Autodesk Inventor part; units mm, degrees
ref_plane "XZ Plane" through (0, 0, 0) normal (0, 1, 0) x (-1, 0, 0)
ref_plane "XY Plane" through (0, 0, 0) normal (0, 0, 1) x (1, 0, 0)
sketch "Sketch1" plane through (0, 0, 0) normal (0, 1, 0) x (-1, 0, 0)
  circle A0 centre (0, 0) radius 9.625
  circle A1 centre (0, 0) radius 7.7
  dimension "d0" = 19.25
  dimension "d1" = 15.4
extrude "Extrusion1" add sketch "Sketch1" along normal blind 1
sketch "Sketch2" plane through (0, 1, 0) normal (0, 1, 0) x (1, 0, 0)
  circle A0 centre (0, 0) radius 9.6436
  line L0 (-2.8579, 4.95) -> (2.8579, 4.95)
  line L1 (2.8579, 4.95) -> (5.7158, 0)
  line L2 (5.7158, 0) -> (2.8579, -4.95)
  line L3 (2.8579, -4.95) -> (-2.8579, -4.95)
  line L4 (-2.8579, -4.95) -> (-5.7158, 0)
  line L5 (-5.7158, 0) -> (-2.8579, 4.95)
  line L6 (0, 0) -> (0, -3.104)
  line L7 (0, 0) -> (3.104, 0) construction
  dimension "d4" = 9.9
  dimension "d5" = 90
extrude "Extrusion2" add sketch "Sketch2" along normal blind 6
sketch "Sketch3" plane through (0, 7, 0) normal (0, 1, 0) x (1, 0, 0)
  circle A0 centre (0, 0) radius 9.6436
  circle A1 centre (0, 0) radius 3.125
  circle A2 centre (0, 0) radius 9.6436
  dimension "d8" = 6.25
  dimension "d9" = 0
extrude "Extrusion3" add sketch "Sketch3" along normal blind 1
fillet "Fillet1" radius 0.2 2 edges at (9.625, 0, 0) (7.7, 0, 0)
sketch "Sketch4" plane through (0, 8, 0) normal (0, 1, 0) x (1, 0, 0)
  circle A0 centre (0, 0) radius 6.5
  circle A1 centre (0, 0) radius 9.6436
  point P0 (5.2807, -5.1416)
  dimension "d15" = 13
extrude "Extrusion4" cut sketch "Sketch4" against normal through all
ref_plane "Work Plane1" through (5, 0, 0) normal (1, 0, 0) x (0, 1, 0)
sketch "Sketch5" plane through (5, 0, 0) normal (1, 0, 0) x (0, 1, 0)
  line L0 (1, 0) -> (1, 4.95)
  line L1 (8, 3.125) -> (8, -3.125)
  line L2 (7, 1.8138) -> (7, -3.5903)
  line L3 (6, 2.0921) -> (6, -3.5903)
  circle A0 centre (6, 0) radius 0.875
  point P0 (0, 0)
  dimension "d19" = 7
  dimension "d20" = 1
  dimension "d21" = 1
  dimension "d22" = 1.75
extrude "Extrusion5" add sketch "Sketch5" along normal blind 4
fillet "Fillet2" radius 0.3 1 edges at (9, 5.125, 0)
mirror "Mirror1" about plane through (0, 0, 0) normal (1, 0, 0) of "Extrusion5", "Fillet2"
sketch "Sketch6" plane through (0, 7, 0) normal (0, -1, 0) x (1, 0, 0)
  circle A0 centre (0, 0) radius 3.125
  line L0 (-5.7158, 0) -> (-2.8579, -4.95)
  line L1 (-2.8579, -4.95) -> (2.8579, -4.95)
  line L2 (2.8579, -4.95) -> (5.7158, 0)
  line L3 (5.7158, 0) -> (2.8579, 4.95)
  line L4 (2.8579, 4.95) -> (-2.8579, 4.95)
  line L5 (-2.8579, 4.95) -> (-5.7158, 0)
extrude "Extrusion6" cut sketch "Sketch6" along normal through all
properties part number "NutRetainer"
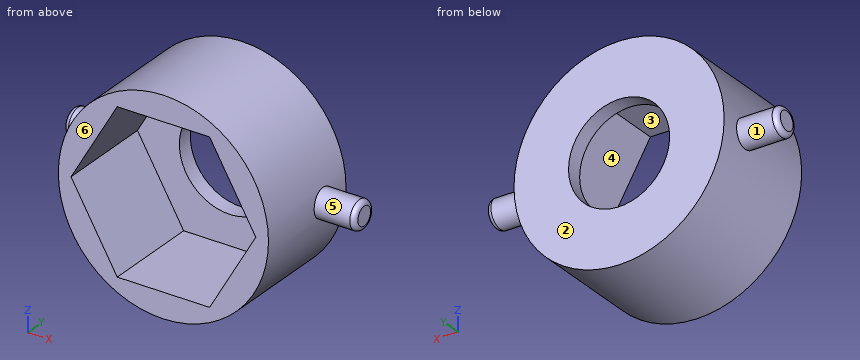
Source: CAD feature listing. Evaluate the final solid. Frame: model axes, mm. Face numbers are marked on the shaded views. A direction names the side the tool comes from. Coordinates: 2 decimals unless noted, no trailing zeros. Order: outer loops, then holes, each group sorted by start corner. A loop starts at its lowest first (then second) coordinate and runs counter-clockwise, first axis right, second up. Notation, with made-up numbers: M 0.25,-19 L 22.25,-19 A19 cw 22.25,-3 Z; hole C 13,6.5 d6. An arc over 180 degrees is marked long. Write each question's results on one line, items separated by ' | '. Start each with the question number.
1. Section B-B, the plane y = 6. Return the cut outline in (x, z) (3 decimals).
2. Reachability of the marked faces 4, 5 and 6 from +Z, -Z, +X, -X, +Y, -Y: full face, straight path, thin tool, end or side. Return the list, or none.
3. Section D-D, the plane z = -4.75. Return the cut outline in (x, y).
4. Material intervals for L1, parallel to Z at x = 0, y = 7.3 (3 decimals); L2, parallel to X at y = 5.25, z = -1.75, sorted ascending.
5. Draft query along Z for the marked faces 1, 2 and 3. Return one class per face: +Z half, -Z half, draft (parallel to the pull), parting line (faces both ways), or undercut.
6. Section A-A, the plane x = 0. Return the cut outline in (y, z) (3 decimals).
7. Pin query (flat end, axial travel): pin 1 (1.5 mm diameter, centred on x = 3.5, y = 4.5, fed in from -Z); pin 2 (1.5 mm diameter, centred on y = 6, z = -2.5, fed in from -X); pin 3 (3 mm diameter, centred on x = -6, y = 5, fed in from +Z). Return the tip coordinate at first contact, or that it passes through.
8. Section C-C, the plane x = -5.25. Return the cut outline in (y, z), then the cut area to 3 significant figures.
Solution:
1) outline: M -9,-0.575 A0.3 ccw -8.7,-0.875 L -6.441,-0.875 A6.5 ccw 6.441,-0.875 L 8.7,-0.875 A0.3 ccw 9,-0.575 L 9,0.575 A0.3 ccw 8.7,0.875 L 6.441,0.875 A6.5 ccw -6.441,0.875 L -8.7,0.875 A0.3 ccw -9,0.575 Z; hole M -5.716,0 L -2.858,-4.95 L 2.858,-4.95 L 5.716,0 L 2.858,4.95 L -2.858,4.95 Z
2) face 4: -Y | face 5: +X | face 6: +Z, -Z, +X, -X, -Y
3) outline: M -4.44,1 L -2.97,1 L -2.97,7 L 2.97,7 L 2.97,1 L 4.44,1 L 4.44,8 L -4.44,8 Z
4) L1: -6.5 to -3.125, 3.125 to 6.5 | L2: -6.26 to -4.71, 4.71 to 6.26
5) face 1: parting line | face 2: draft | face 3: undercut
6) outline: M 1,-6.5 L 8,-6.5 L 8,-3.125 L 7,-3.125 L 7,-4.95 L 1,-4.95 Z; M 1,4.95 L 7,4.95 L 7,3.125 L 8,3.125 L 8,6.5 L 1,6.5 Z
7) pin 1: z = -5.89 | pin 2: x = -6.26 | pin 3: z = 4.69
8) outline: M 1,-3.83 L 8,-3.83 L 8,3.83 L 1,3.83 L 1,0.81 L 7,0.81 L 7,-0.81 L 1,-0.81 Z | area: 44.0 mm²
